Design review of the part built by this model. Coordinates are the model's own, in mm. Give positions to 0.01 mm unless a question says otherwise; leave off trailing zeros. Write each loop counter-clockwise with the first axis right and the second up, starting at its lowest first coordinate (ties: lowest second). Pieces come first, ordered by that corner, then holes. Notation, with made-up numbers: (78, 66) - (107, 66) arc R12 ccw to (107, 73) - close; hole circle Ø4 at (1, 59). An arc over 180 degrees is marked (long way). Use a Markdown table: item, result. Add a question column.
```python
from build123d import *

# Parameters (mm, degrees)
F0_W     = 24
F0_H     = 24
F0_R     = 1.6
F1_DEPTH = 3
F2_SIZE  = 4
F3_COUNT = 4


with BuildPart() as f1:
    # F0 (on Top) → F1 (new body)
    with BuildSketch(Plane.XY):
        with Locations((13, 13)):
            Rectangle(F0_W, F0_H)
        with Locations((16, 10)):
            Circle(F0_R, mode=Mode.SUBTRACT)
        with Locations((10, 16)):
            Circle(F0_R, mode=Mode.SUBTRACT)
    extrude(amount=F1_DEPTH)

    # F2
    f2_edges = [f1.edges().sort_by_distance(p)[0] for p in [
        (1, 1, 1.5),
    ]]
    chamfer(f2_edges, length=F2_SIZE)

    # F3: F1 ×4 about axis
    f3_axis = Axis((25, 25, 1.5), (0, 0, -1))


with BuildPart() as f1_1:
    add(f1.part)
    for i in range(1, F3_COUNT):
        add(f1.part.rotate(f3_axis, i * 360 / F3_COUNT))


solid = f1_1.part
```
(1) For line 1 along X through (y, z) = (40, 1.5); line 2 along X through (y, z) = (34, 0.75), list the stretches that pass through material, from the lowest coordinate up.
(2) Add section A-A (z = 1.95). Count the separate pieces of the cut face and the enclosed holes in it, and give its area (3 significant figures).
(3) Insertion check: pin 1 (2.5 mm diameter, centred on x = 40, y = 34, fed in from -Z). The pin has a flat end and moves straight along its axis. Give the tip position at first contact, or say it passes through.
(4) Mouldability with a two-part tool opening along X and no side actions: class faces 1 (the face through (25, 1, 1)), 2 (the face through (14.4, 10.07, 1.48)), 3 (the face through (49, 25, 1)) as +X half, -X half, draft (parallel to the pull), parting line (faces both ways), or undercut.
(5) Add section B-B (y = 10). State the section outline as (x, z) points, and give its area (3 significant figures).
Answers follow:
| question | item | result |
|---|---|---|
| 1 | line 1 | 1 to 14.4, 17.6 to 32.4, 35.6 to 49 |
| 1 | line 2 | 1 to 8.4, 11.6 to 38.4, 41.6 to 49 |
| 2 | separate pieces | 1 |
| 2 | enclosed holes | 8 |
| 2 | area | 2,210 mm^2 |
| 3 | pin 1 | through |
| 4 | face 1 | draft |
| 4 | face 2 | undercut |
| 4 | face 3 | +X half |
| 5 | outline | (1, 0) - (14.4, 0) - (14.4, 3) - (1, 3) - close; (17.6, 0) - (32.4, 0) - (32.4, 3) - (17.6, 3) - close; (35.6, 0) - (49, 0) - (49, 3) - (35.6, 3) - close |
| 5 | area | 125 mm^2 |
